```python
from build123d import *

# Parameters (mm, degrees)
SKETCH1_R               = 16.5
SKETCH1_R_2             = 12.5
BOSS_EXTRUDE1_DEPTH     = 7.4
SKETCH6_R               = 19.5
SKETCH6_R_2             = 12.5
BOSS_EXTRUDE2_DEPTH     = 3.6
SKETCH12_R              = 12.5
SKETCH12_R_2            = 1.5
BOSS_EXTRUDE4_DEPTH     = 18.4
CHAMFER3_SIZE           = 3.6
CUT_EXTRUDE1_DEPTH      = 35.662660025
CUT_EXTRUDE1_DEPTH_BACK = 35.662660025
SKETCH14_R              = 3


with BuildPart() as part:
    # Sketch1 → Boss-Extrude1 (new, symmetric)
    with BuildSketch(Plane.XY):
        Circle(SKETCH1_R)
        Circle(SKETCH1_R_2, mode=Mode.SUBTRACT)
    extrude(amount=BOSS_EXTRUDE1_DEPTH, both=True)

    # Sketch6 → Boss-Extrude2 (add)
    with BuildSketch(Plane.XY.offset(7.4)):
        Circle(SKETCH6_R)
        Circle(SKETCH6_R_2, mode=Mode.SUBTRACT)
    boss_extrude2 = extrude(amount=BOSS_EXTRUDE2_DEPTH)

    # Mirror1: Boss-Extrude2 across plane
    add(boss_extrude2.mirror(Plane.XY))

    # Sketch12 → Boss-Extrude4 (add)
    with BuildSketch(Plane.XY.offset(11)):
        with Locations(Location((0, 0, 0), (0, 0, 180))):
            Circle(SKETCH12_R)
        Circle(SKETCH12_R_2, mode=Mode.SUBTRACT)
    extrude(amount=-BOSS_EXTRUDE4_DEPTH)

    # Chamfer3
    chamfer3_edges = [part.edges().sort_by_distance(p)[0] for p in [
        (-12.5, 0, -7.4),
    ]]
    chamfer(chamfer3_edges, length=CHAMFER3_SIZE - 0.0001)  # a hair under: the kernel refuses the full size

    # Fillet3: read off the stored shape, not the designer's step
    # Fillet3 outline → Fillet3 (revolve, cut)
    with BuildSketch(Plane.XZ):
        with BuildLine():
            Line((11.914213562, -11), (13.328427125, -11))
            ThreePointArc((13.328427125, -11), (12.56306026, -10.847759065), (11.914213562, -10.414213562))
            Line((11.914213562, -10.414213562), (11.914213562, -11))
        make_face()
    revolve(axis=Axis((0, 0, 0), (0, 0, 1)), mode=Mode.SUBTRACT)

    # Fillet3 2 outline → Fillet3 2 (revolve)
    with BuildSketch(Plane.XZ):
        with BuildLine():
            ThreePointArc((8.071572875, -7.4), (8.83693974, -7.552240935), (9.485786438, -7.985786438))
            Line((9.485786438, -7.985786438), (9.485786438, -7.4))
            Line((9.485786438, -7.4), (8.071572875, -7.4))
        make_face()
    revolve(axis=Axis((0, 0, 0), (0, 0, 1)))

    # Sketch14 → Cut-Extrude1 (cut, two sides: drawn at the far end of the back side and taken through both)
    with BuildSketch(Plane.XY.offset(-10).offset(-CUT_EXTRUDE1_DEPTH_BACK)):
        Circle(SKETCH14_R)
    extrude(amount=CUT_EXTRUDE1_DEPTH + CUT_EXTRUDE1_DEPTH_BACK, mode=Mode.SUBTRACT)


solid = part.part
```
For this review, take the finished solid that the model builds, in its own axes (mm). A direction names the side the tool comes from. Coordinates: 2 decimals unless noted, no trailing zeros. Loops run counter-clockwise (first coordinate to the right, second up) from the corner with the lowest first, then second, coordinate; pieces in that order, holes last.
1. For line 1 (Z direction, x = -1.5, y = -16.5); line 2 (Y direction, x = 0, z = 5); line 3 (Z direction, x = 10, y = 6.5), list the stretches that pass through material, from the lowest coordinate up.
2. Add section C-C, the plane z = 9.5. Give the boundary of the cut face in (x, y).
3. Mouldability with a two-part tool opening along X and no side actions: class faces 3 (the flat face through (0, 4, 11)), 4 (the flat face through (-3.5, -0.1, -7.4)), 5 (the conical face through (4.45, 8.55, -8.14)), 6 (the cylindrical face through (-2.539, 19.334, 9.175)) as +X half, -X half, draft (parallel to the pull), parting line (faces both ways), or undercut.
4. For faces 1 (the flat face through (-15, 9, -7.4)), 2 (the cylindrical face through (-2.539, 19.334, -9.175)), list the 3-axis set-ups (+Z, -Z, +X, -X, +Y, -Y) from which the entire face can be reached by the end or side of a thin tool; tool diameter is ignored.
5. Add section D-D, the plane x = 14. Give the boundary of the cut face in (y, z), then the cut area to 3 significant figures.
6. Insertion check: P1, Ø3, axis at x = -6, z = 5, coming from the +Y side; P2, Ø10, axis at y = -6, z = 5.5, coming from the -X side; P3, Ø4, axis at y = -4, z = -4, coming from the +X side; P4, Ø5, axis at x = 0, y = 0, coming from the -Z side. Each pin has a flat end and moves straight along its axis. Give the tip position at first contact, or say it passes through.
Result:
1. line 1: z = -11 to -7.4, 7.4 to 11
1. line 2: y = -16.5 to -3, 3 to 16.5
1. line 3: z = -10.43 to 11
2. outline: circle Ø39 at (0, 0); hole circle Ø6 at (0, 0)
3. face 3: draft
3. face 4: undercut
3. face 5: undercut
3. face 6: parting line
4. face 1: none
4. face 2: +Z, -Z
5. outline: (-13.57, -11) - (13.57, -11) - (13.57, -7.4) - (8.73, -7.4) - (8.73, 7.4) - (13.57, 7.4) - (13.57, 11) - (-13.57, 11) - (-13.57, 7.4) - (-8.73, 7.4) - (-8.73, -7.4) - (-13.57, -7.4) - close
5. area: 454 mm2
6. P1: stops at y = 15.87
6. P2: stops at x = -19.45
6. P3: stops at x = 16.38
6. P4: passes through
